Answer from the drawing. Dimensions are ordinates in mm from the lowest x, y and z of the part. A direction names the side the tool comes from. Give positions to 0.01 mm unless a question says otherwise; leave off trailing zeros. Loops run counter-clockwise (first coordinate to the right, second up) from the corner with the lowest first, then second, coordinate; pieces in that order, holes last.
Item 1: Section C-C, the plane y = 11.5 is taken. Give the vertices of the cut face in (x, z), and give its area (3 significant figures).
Item 2: Section B-B, the plane z = 1 is taken. Give the vertices of the cut face in (x, y), and give its area (3 significant figures).
Item 3: A tool of negligible diameter and unlimited length cuts with its end or side. For the marked faces 4 and 5, from which of +Z, -Z, +X, -X, +Y, -Y can it reach the whole face along a straight path? Write none if from no direction.
Item 4: Consider line 1 along X through (y, z) = (8.5, 2.5); line 2 along Z through (x, y) = (5, 9); line 3 along X through (y, z) = (2, 6). Determine where each line is inside the solid, lowest interval first.
Item 5: The mould has two halves that part along X. Classify the marked faces 1, 2 and 3: pulls with the +X half, pulls with the -X half, needs draft (parallel to the pull), parting line crosses it, or undercut.
Item 6: Section D-D, the plane x = 23 is taken. Give the vertices of the cut face in (y, z), and give its area (3 significant figures).
Item 7: Section A-A, the plane y = 4 is taken. Give the vertices of the cut face in (x, z).
Item 8: Each of these flat-tipped pins is pushed along its axis until it touches: pin 1 Ø5.5 at (x, z) = (5, 5) entering from +Y; pin 2 Ø6 at (y, z) = (25.5, 6.5) entering from -X; pin 3 Ø3.5 at (x, z) = (5, 5) entering from -Y. Where does it stop, or does it pass through?
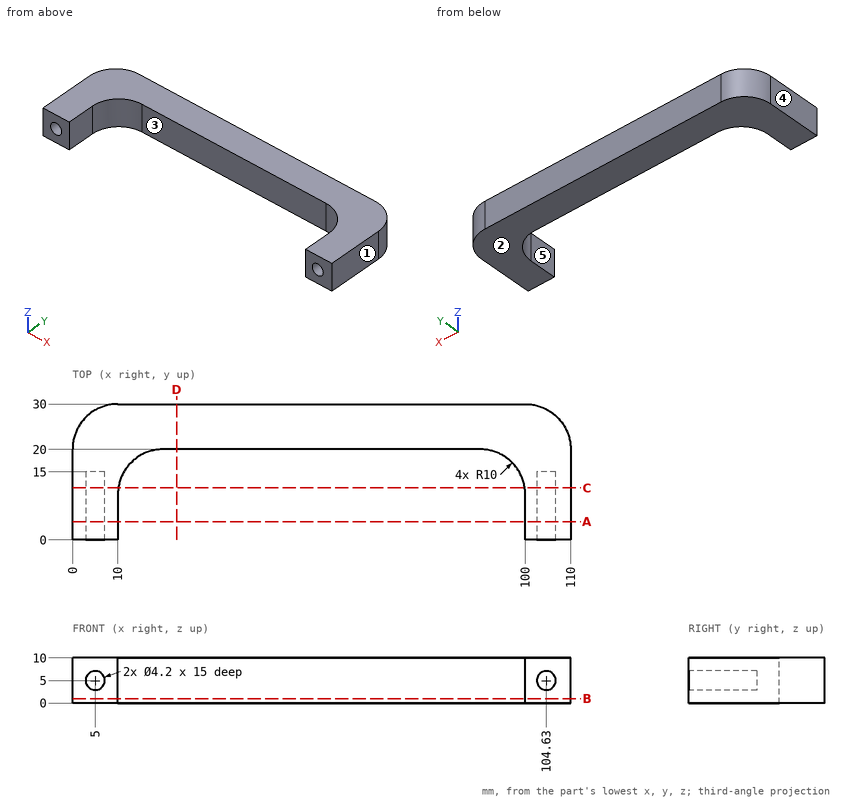
Worked answers:
1. outline: (0, 0) - (10.11, 0) - (10.11, 10) - (0, 10) - close; (99.89, 0) - (110, 0) - (110, 10) - (99.89, 10) - close; hole circle Ø4.2 at (5, 5); hole circle Ø4.2 at (104.63, 5)
1. area: 175 mm2
2. outline: (0, 0) - (10, 0) - (10, 10) arc R10 cw to (20, 20) - (90, 20) arc R10 cw to (100, 10) - (100, 0) - (110, 0) - (110, 20) arc R10 ccw to (100, 30) - (10, 30) arc R10 ccw to (0, 20) - close
2. area: 1,500 mm2
3. face 4: +Z, -Z, -X, +Y, -Y
3. face 5: +Z, -Z, -Y
4. line 1: x = 0 to 10, 100 to 110
4. line 2: z = 0 to 2.9, 7.1 to 10
4. line 3: x = 0 to 3.15, 6.85 to 10, 100 to 102.78, 106.48 to 110
5. face 1: pulls with the +X half
5. face 2: needs draft
5. face 3: undercut
6. outline: (20, 0) - (30, 0) - (30, 10) - (20, 10) - close
6. area: 100 mm2
7. outline: (0, 0) - (10, 0) - (10, 10) - (0, 10) - close; (100, 0) - (110, 0) - (110, 10) - (100, 10) - close; hole circle Ø4.2 at (5, 5); hole circle Ø4.2 at (104.63, 5)
8. pin 1: stops at y = 29.74
8. pin 2: stops at x = 0.32
8. pin 3: stops at y = 15
